Part model, mm, in its own coordinate system. Give positions to 0.01 mm unless a question says otherwise; leave off trailing zeros. Write item = value, one per line. Start each with the question number.
(1) Saw through at A-A, the plane y = 1.3. State how many separate pieces and enclosed holes the cut face has, then the cut area to 3 significant figures.
(2) Probe line 1 along X through (y, z) = (1.55, -317.5); line 2 along X through (y, z) = (1.05, -163); line 3 along Z through (x, y) = (-1.5, 1.85). List the from-to ranges inside material, lowest first. Write a range as from..to.
(3) Flat gauge pin, fed straight in: pin 1 (3 mm diameter, centred on x = -12.7, z = -165.1, fed in from -Y). Where does the tip first touch, or does it go through?
Autodesk Inventor part; units mm, degrees
ref_plane "YZ Plane" through (0, 0, 0) normal (1, 0, 0) x (0, 1, 0)
ref_plane "XZ Plane" through (0, 0, 0) normal (0, 1, 0) x (-1, 0, 0)
ref_plane "XY Plane" through (0, 0, 0) normal (0, 0, 1) x (1, 0, 0)
sketch "Sketch1" plane through (0, 0, 0) normal (0, 1, 0) x (-1, 0, 0)
  line L0 (3.175, 0) -> (22.225, 0)
  line L1 (25.4, -3.175) -> (25.4, -403.225)
  line L2 (22.225, -406.4) -> (3.175, -406.4)
  line L3 (0, -403.225) -> (0, -3.175)
  arc A0 (25.4, -3.175) -> (22.225, 0) centre (22.225, -3.175) ccw
  arc A1 (3.175, 0) -> (0, -3.175) centre (3.175, -3.175) ccw
  arc A2 (22.225, -406.4) -> (25.4, -403.225) centre (22.225, -403.225) ccw
  arc A3 (0, -403.225) -> (3.175, -406.4) centre (3.175, -403.225) ccw
  circle A4 centre (12.7, -12.7) radius 2.54
  circle A5 centre (12.7, -25.4) radius 2.54
  circle A6 centre (12.7, -38.1) radius 2.54
  circle A7 centre (12.7, -50.8) radius 2.54
  circle A8 centre (12.7, -63.5) radius 2.54
  circle A9 centre (12.7, -76.2) radius 2.54
  circle A10 centre (12.7, -88.9) radius 2.54
  circle A11 centre (12.7, -101.6) radius 2.54
  circle A12 centre (12.7, -114.3) radius 2.54
  circle A13 centre (12.7, -127) radius 2.54
  circle A14 centre (12.7, -139.7) radius 2.54
  circle A15 centre (12.7, -152.4) radius 2.54
  circle A16 centre (12.7, -165.1) radius 2.54
  circle A17 centre (12.7, -177.8) radius 2.54
  circle A18 centre (12.7, -190.5) radius 2.54
  circle A19 centre (12.7, -203.2) radius 2.54
  circle A20 centre (12.7, -215.9) radius 2.54
  circle A21 centre (12.7, -228.6) radius 2.54
  circle A22 centre (12.7, -241.3) radius 2.54
  circle A23 centre (12.7, -254) radius 2.54
  circle A24 centre (12.7, -266.7) radius 2.54
  circle A25 centre (12.7, -279.4) radius 2.54
  circle A26 centre (12.7, -292.1) radius 2.54
  circle A27 centre (12.7, -304.8) radius 2.54
  circle A28 centre (12.7, -317.5) radius 2.54
  circle A29 centre (12.7, -330.2) radius 2.54
  circle A30 centre (12.7, -342.9) radius 2.54
  circle A31 centre (12.7, -355.6) radius 2.54
  circle A32 centre (12.7, -368.3) radius 2.54
  circle A33 centre (12.7, -381) radius 2.54
  circle A34 centre (12.7, -393.7) radius 2.54
  point P0 (0, 0)
  dimension "d0" = 25.4
  dimension "d1" = 406.4
  dimension "d2" = 3.175
  dimension "d3" = 3.175
  dimension "d4" = 12.7
  dimension "d5" = 5.08
  dimension "d6" = 12.7
  dimension "d9" = 12.7
extrude "Extrusion1" add sketch "Sketch1" along normal blind 3.175
properties part number "ELEV_016_SUPBAR1" material "Aluminum 6061"
Results list:
q1.separate_pieces = 1
q1.enclosed_holes = 31
q1.area = 9,690 mm^2
q2.line_1 = -25.4..-15.24, -10.16..0
q2.line_2 = -25.4..-14.13, -11.27..0
q2.line_3 = -405.92..-0.48
q3.pin_1 = through
